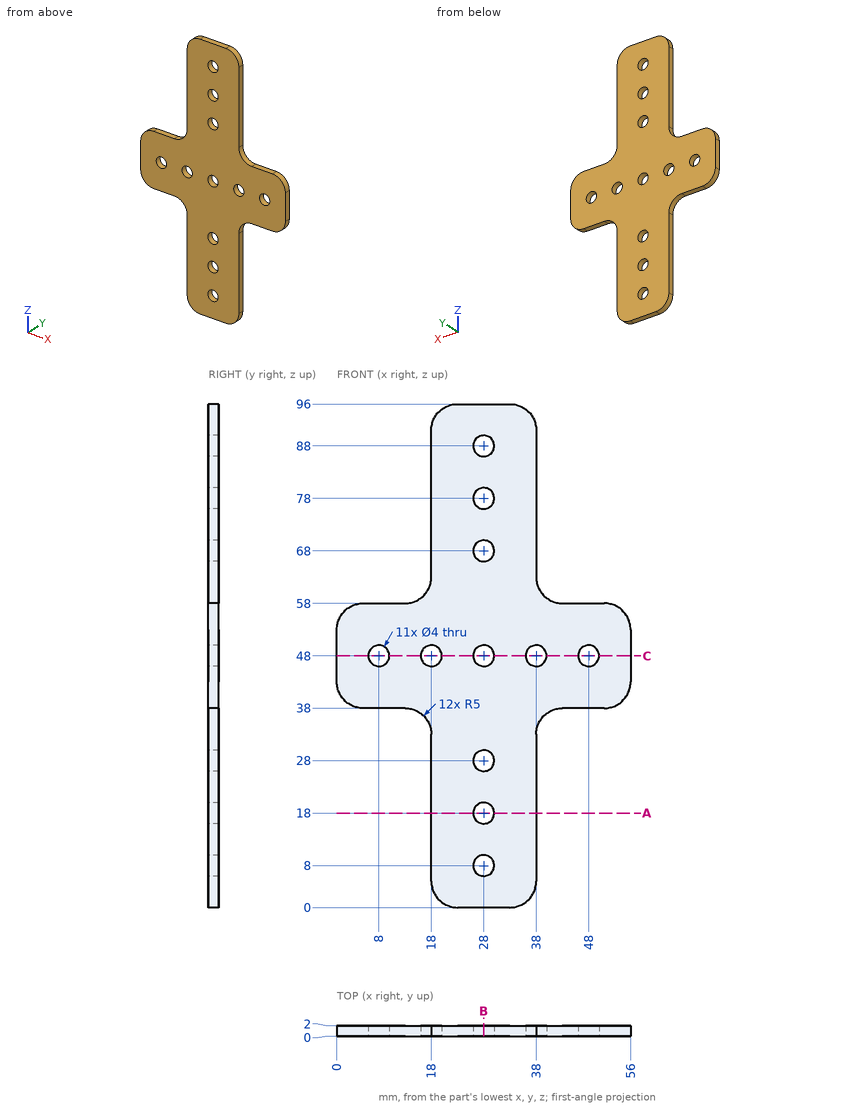
For this review, use the dimensioned drawing (mm, ordinates from the lowest corner) and the shaded views. Give positions to 0.01 mm unless a question says otherwise; leave off trailing zeros. Loops run counter-clockwise (first coordinate to the right, second up) from the corner with the lowest first, then second, coordinate; pieces in that order, holes last.
Item 1: Insertion check: pin 1 (0.6 mm diameter, centred on x = 9.5, y = 0.5, fed in from +Z); pin 2 (2.5 mm diameter, centred on x = 28, z = 8, fed in from +Y); pin 3 (5 mm diameter, centred on x = 38, z = 48, fed in from -Y); pin 4 (1 mm diameter, centred on y = 0.5, z = 54.5, fed in from +X). Each pin has a flat end and moves straight along its axis. Give the tip position at first contact, or say it passes through.
Item 2: Take a section at B-B, the plane x = 28. Give the number of separate pieces and of enclosed holes in the cut face, and give its area (3 significant figures).
Item 3: Take a section at A-A, the plane z = 18. State the section outline as (x, y) points, and give its area (3 significant figures).
Item 4: For line 1 along X through (y, z) = (0.65, 48); line 2 along X through (y, z) = (1.75, 78); line 3 along X through (y, z) = (1, 73.5), list the stretches that pass through material, from the lowest coordinate up.
Item 5: Take a section at C-C, the plane z = 48. State the section outline as (x, y) points.
Calculated:
1. pin 1: stops at z = 58
1. pin 2: passes through
1. pin 3: stops at y = 0
1. pin 4: stops at x = 55.9
2. separate pieces: 8
2. enclosed holes: 0
2. area: 136 mm2
3. outline: (18, 0) - (26, 0) - (26, 2) - (18, 2) - close; (30, 0) - (38, 0) - (38, 2) - (30, 2) - close
3. area: 32.0 mm2
4. line 1: x = 0 to 6, 10 to 16, 20 to 26, 30 to 36, 40 to 46, 50 to 56
4. line 2: x = 18 to 26, 30 to 38
4. line 3: x = 18 to 38
5. outline: (0, 0) - (6, 0) - (6, 2) - (0, 2) - close; (10, 0) - (16, 0) - (16, 2) - (10, 2) - close; (20, 0) - (26, 0) - (26, 2) - (20, 2) - close; (30, 0) - (36, 0) - (36, 2) - (30, 2) - close; (40, 0) - (46, 0) - (46, 2) - (40, 2) - close; (50, 0) - (56, 0) - (56, 2) - (50, 2) - close
